from build123d import *

# Parameters (mm, degrees)
SKETCH1_R           = 22.5
SKETCH1_R_2         = 12.5
BOSS_EXTRUDE1_DEPTH = 20
FILLET1_R           = 3
FILLET2_R           = 1


with BuildPart() as part:
    # Sketch1 → Boss-Extrude1 (new, symmetric)
    with BuildSketch(Plane.XY):
        Circle(SKETCH1_R)
        Circle(SKETCH1_R_2, mode=Mode.SUBTRACT)
    extrude(amount=BOSS_EXTRUDE1_DEPTH, both=True)

    # Fillet1
    fillet1_edges = [part.edges().sort_by_distance(p)[0] for p in [
        (-22.5, 0, 20),
        (-22.5, 0, -20),
    ]]
    fillet(fillet1_edges, radius=FILLET1_R)

    # Fillet2
    fillet2_edges = [part.edges().sort_by_distance(p)[0] for p in [
        (-12.5, 0, -20),
        (-12.5, 0, 20),
    ]]
    fillet(fillet2_edges, radius=FILLET2_R)


solid = part.part
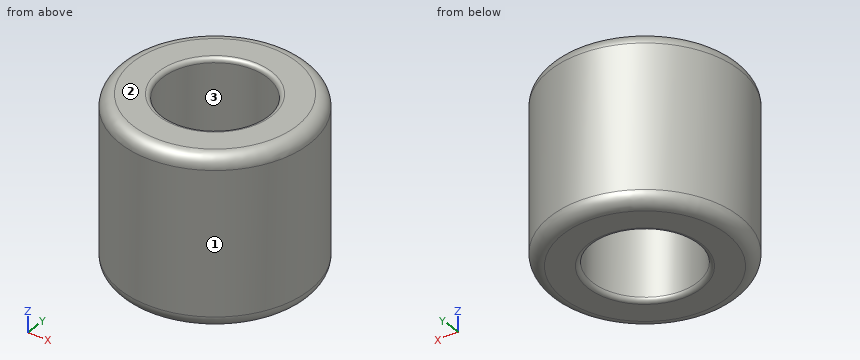
The listing builds one solid part. Answer for the finished solid, in the listing's coordinates (mm). Face numbers are marked on the shaded views. Coordinates: 2 decimals unless noted, no trailing zeros. Write each loop counter-clockwise with the first axis right and the second up, starting at its lowest first coordinate (ties: lowest second). Pieces come first, ordered by that corner, then holes. Notation, with made-up numbers: M 54.5,73 L 77.5,73 A23 cw 77.5,107 Z; hole C -6,51 d3. An arc over 180 degrees is marked long. Use one line per item in the form item = value.
Item 1: The mould has two halves that part along Y. Classify the marked faces 1, 2 and 3: released by +Y, released by -Y, zero draft, split by the parting line, or undercut.
Model answer:
face_1 = split by the parting line
face_2 = zero draft
face_3 = undercut
Item 2: Find section C-C, the plane z = 9.5. Give the vertices of the cut face in (x, y), plus the area to 3 significant figures.
Model answer:
outline = C 0,0 d45; hole C 0,0 d25
area = 1,100 mm2
Item 3: Given P1, Ø12, axis at x = 6, z = -3, coming from the -Y side; P2, Ø12, axis at x = -8, z = 16, coming from the +Y side; P3, Ø1, axis at x = -17, y = 14, coming from the +Z side, each flat-ended and moving along its own axis, determine where each tip first touches the part or whether it passes through.
Model answer:
P1 = -22.5
P2 = 22.41
P3 = 19.22
Item 4: Find section A-A, the plane y = 0. Give the vertices of the cut face in (x, z), plus the area to 3 significant figures.
Model answer:
outline = M -22.5,-17 A3 ccw -19.5,-20 L -13.5,-20 A1 ccw -12.5,-19 L -12.5,19 A1 ccw -13.5,20 L -19.5,20 A3 ccw -22.5,17 Z; M 12.5,-19 A1 ccw 13.5,-20 L 19.5,-20 A3 ccw 22.5,-17 L 22.5,17 A3 ccw 19.5,20 L 13.5,20 A1 ccw 12.5,19 Z
area = 791 mm2
Item 5: Find the intervals of material crossed by probe 1 along Y at (x, z) = (0, 11); probe 2 along X at (y, z) = (-10.5, -16); probe 3 along Y at (x, z) = (-5, -17), in increasing order.
Model answer:
probe_1 = -22.5 to -12.5, 12.5 to 22.5
probe_2 = -19.9 to -6.78, 6.78 to 19.9
probe_3 = -21.94 to -11.46, 11.46 to 21.94
